Read the model definition and answer for the solid it produces. Units are mm, in the model's axes. A direction names the side the tool comes from. Coordinates: 2 decimals unless noted, no trailing zeros. Order: outer loops, then holes, each group sorted by start corner. A loop starts at its lowest first (then second) coordinate and runs counter-clockwise, first axis right, second up. Notation, with made-up numbers: M -3,76.25 L 1,76.25 A11 ccw 1,93.25 Z; hole C -16,17.5 d4. An arc over 180 degrees is marked long. Use a Markdown table: item, result. Add a question column.
1) Find section A-A on z = -14.75. Write down the section's boundary in (x, y) (3 decimals).
2) Find section B-B on y = 506.5. Write down the section's boundary in (x, z) (3 decimals).
3) For faces 4 (the face through (-26, 479, -25.4)), 5 (the face through (-25, 479, -22.225)), determine the directions among +Z, -Z, +X, -X, +Y, -Y from which every point of the face is accessible in a straight line to the end or side of a thin tool.
4) Find the intervals of material crossed by probe 1 along X at (y, z) = (169, -19) (3 decimals); probe 2 along Z at (x, y) = (-44.5, 298.5) (3 decimals); probe 3 along Y at (x, z) = (-1.5, -24), in increasing order. Write a range as [from, to].
5) The mould has two halves that part along X. Classify faces 1 (the face through (-47.625, 479, -13)), 2 (the face through (-50.8, 479, -13)), 3 (the face through (-25.52, 828.74, -2.29)): released by +X, released by -X, zero draft, split by the parting line, or undercut.
6) Each of these flat-tipped pins is pushed along its axis until it touches: pin 1 Ø15 at (y, z) = (581, -14.5) entering from +X; pin 2 Ø10 at (x, z) = (-8.5, -9) entering from -Y. Where does it stop, or does it pass through?
7) Find section C-C on x = -33. Write down the section's boundary in (y, z) (3 decimals).
Autodesk Inventor part; units mm, degrees
ref_plane "YZ Plane" through (0, 0, 0) normal (1, 0, 0) x (0, 1, 0)
ref_plane "XZ Plane" through (0, 0, 0) normal (0, 1, 0) x (-1, 0, 0)
ref_plane "XY Plane" through (0, 0, 0) normal (0, 0, 1) x (1, 0, 0)
sketch "Sketch1" plane through (0, 0, 0) normal (0, 1, 0) x (-1, 0, 0)
  line L0 (0, 0) -> (50.8, 0)
  line L1 (50.8, 0) -> (50.8, -25.4)
  line L2 (50.8, -25.4) -> (0, -25.4)
  line L3 (0, -25.4) -> (0, 0)
  line L4 (47.625, -22.225) -> (47.625, -3.175)
  line L5 (47.625, -3.175) -> (3.175, -3.175)
  line L6 (3.175, -3.175) -> (3.175, -22.225)
  line L7 (3.175, -22.225) -> (47.625, -22.225)
  dimension "d0" = 50.8
  dimension "d1" = 25.4
  dimension "d2" = 3.175
extrude "Extrusion1" add sketch "Sketch1" along normal blind 886.206
sketch "Sketch2" plane through (-50.8, 0, 0) normal (0, 0, 1) x (1, 0, 0)
  line L0 (50.8, 0) -> (0, 0)
  line L1 (50.8, 0) -> (50.8, 886.206)
  line L2 (0, 886.206) -> (50.8, 886.206)
  line L3 (0, 0) -> (0, 886.206)
  line L4 (0, 0) -> (50.8, 0)
  line L5 (50.8, 0) -> (0, 56.4191)
  line L6 (0, 56.4191) -> (50.8, 56.4191)
  line L7 (50.8, 56.4191) -> (50.8, 0)
  line L8 (50.8, 0) -> (0, 0)
  line L9 (0, 0) -> (0, 56.4191)
  line L10 (0, 56.4191) -> (50.8, 0)
  line L11 (0, 56.4191) -> (21.859, 0)
  line L12 (47.625, 0) -> (3.175, 0)
  dimension "d5" = 48
extrude "Extrusion2" cut sketch "Sketch2" against normal blind 914.4 contours L0 L11 L5 | L11 L0 L3
sketch "Sketch3" plane through (-50.8, 886.206, 0) normal (0, 0, 1) x (1, 0, 0)
  line L0 (0, -829.7869) -> (50.8, -886.206)
  line L1 (50.8, -886.206) -> (50.8, 0)
  line L2 (0, 0) -> (50.8, 0)
  line L3 (0, -829.7869) -> (0, 0)
  line L4 (0, -829.7869) -> (50.8, -886.206)
  line L5 (0, -829.7869) -> (50.8, -778.9869)
  line L6 (50.8, -886.206) -> (50.8, 0)
  line L7 (0, -829.7869) -> (0, 0)
  line L8 (50.8, -886.206) -> (0, -886.206)
  line L9 (0, -886.206) -> (0, -923.3654)
  line L10 (0, -923.3654) -> (50.8, -923.3654)
  line L11 (50.8, -923.3654) -> (50.8, -886.206)
  dimension "d8" = 93
extrude "Extrusion3" cut sketch "Sketch3" against normal blind 25.4 contours L5 L1 L0
sketch "Sketch4" plane through (-50.8, 886.206, 0) normal (0, 0, 1) x (1, 0, 0)
  line L0 (0, -829.7869) -> (50.8, -778.9869)
  line L1 (50.8, -778.9869) -> (50.8, 0)
  line L2 (0, 0) -> (50.8, 0)
  line L3 (0, -829.7869) -> (0, 0)
  line L4 (0, 0) -> (50.8, 0)
  line L5 (0, 0) -> (50.8, 0)
  line L6 (50.8, 0) -> (50.8, -221.7928)
  line L7 (50.8, -221.7928) -> (0, -221.7928)
  line L8 (0, -221.7928) -> (0, 0)
  line L9 (0, -829.7869) -> (0, 0)
  line L10 (0, 0) -> (50.8, -50.8)
  line L11 (50.8, 0) -> (0, 0)
  line L12 (0, 0) -> (0, -56.4191)
  line L13 (0, -56.4191) -> (50.8, -56.4191)
  line L14 (50.8, -56.4191) -> (50.8, 0)
  point P0 (50.8, -886.206)
  dimension "d11" = 221.7928
  dimension "d12" = 45
  dimension "d13" = 56.4191
extrude "Extrusion4" cut sketch "Sketch4" against normal blind 25.4 contours L2 L1 L10
sketch "Sketch8" plane through (-50.8, 56.4191, 0) normal (0, 0, 1) x (1, 0, 0)
  line L0 (50.8, 778.9869) -> (0, 829.7869)
  line L1 (0, 0) -> (0, 829.7869)
  line L2 (0, 0) -> (50.8, 50.8)
  line L3 (50.8, 50.8) -> (50.8, 778.9869)
  line L4 (0, 797.6016) -> (50.8, 746.8016)
  point P0 (50.8, -56.4191)
  dimension "d24" = 22.7584
extrude "Extrusion8" cut sketch "Sketch8" against normal blind 25.4 contours L3 L4 L1 L0
sketch "Sketch9" plane through (-50.8, 56.4191, 0) normal (0, 0, 1) x (1, 0, 0)
  line L0 (50.8, 746.8016) -> (0, 797.6016)
  line L1 (0, 0) -> (0, 797.6016)
  line L2 (0, 0) -> (50.8, 50.8)
  line L3 (50.8, 50.8) -> (50.8, 746.8016)
  line L4 (0, 0) -> (0, 797.6016)
  line L5 (0, 58.228) -> (50.8, 109.028)
  line L6 (50.8, 50.8) -> (50.8, 746.8016)
  line L7 (0, 0) -> (50.8, 50.8)
  point P0 (50.8, -56.4191)
  dimension "d27" = 41.1734
extrude "Extrusion9" cut sketch "Sketch9" against normal blind 25.4 contours L3 L2 L1 L5
properties part number "AngleBrace.ver1-1111-2020" material "Aluminum 6061"
Check result:
| question | item | result |
|---|---|---|
| 1 | outline | M -50.8,114.647 L -47.625,117.822 L -47.625,850.846 L -50.8,854.021 Z; M -3.175,162.272 L 0,165.447 L 0,803.221 L -3.175,806.396 Z |
| 2 | outline | M -50.8,-25.4 L 0,-25.4 L 0,0 L -50.8,0 Z; hole M -47.625,-22.225 L -3.175,-22.225 L -3.175,-3.175 L -47.625,-3.175 Z |
| 3 | face 4 | -Z, +X, -X, +Y, -Y |
| 3 | face 5 | +Y, -Y |
| 4 | probe 1 | x = [-50.8, -47.625], [-3.175, 0] |
| 4 | probe 2 | z = [-25.4, -22.225], [-3.175, 0] |
| 4 | probe 3 | y = [163.95, 804.72] |
| 5 | face 1 | undercut |
| 5 | face 2 | released by -X |
| 5 | face 3 | released by +X |
| 6 | pin 1 | stops at x = 0 |
| 6 | pin 2 | passes through |
| 7 | outline | M 132.447,-25.4 L 836.221,-25.4 L 836.221,-22.225 L 132.447,-22.225 Z; M 132.447,-3.175 L 836.221,-3.175 L 836.221,0 L 132.447,0 Z |
